Design review of the part built by this model. Coordinates are the model's own, in mm. Round coordinates to 2 decimals unless told otherwise and drop trailing zeros. Order: outer loops, then holes, each group sorted by start corner. A loop starts at its lowest first (then second) coordinate and runs counter-clockwise, first axis right, second up.
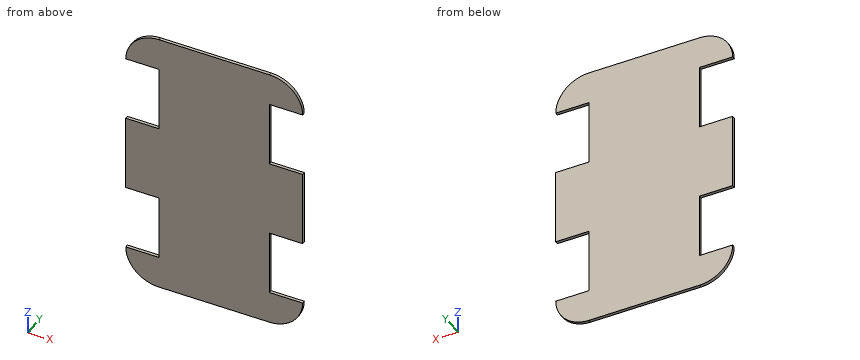
from build123d import *

# Parameters (mm, degrees)
BOSS_EXTRUDE1_DEPTH = 2.8


with BuildPart() as part:
    # Sketch1 → Boss-Extrude1 (new body)
    with BuildSketch(Plane(origin=(0, 0, 0), x_dir=(1, 0, 0), z_dir=(0, 1, 0))):
        with BuildLine():
            Line((0, 30), (30, 30))
            Line((30, 30), (30, 90))
            Line((30, 90), (0, 90))
            Line((0, 90), (0, 160))
            Line((0, 160), (30, 160))
            Line((30, 160), (30, 220))
            Line((30, 220), (0, 220))
            ThreePointArc((0, 220), (8.786796564, 241.213203436), (30, 250))
            Line((30, 250), (130, 250))
            ThreePointArc((130, 250), (151.213203436, 241.213203436), (160, 220))
            Line((160, 220), (130, 220))
            Line((130, 220), (130, 160))
            Line((130, 160), (160, 160))
            Line((160, 160), (160, 90))
            Line((160, 90), (130, 90))
            Line((130, 90), (130, 30))
            Line((130, 30), (160, 30))
            ThreePointArc((160, 30), (151.213203436, 8.786796564), (130, 0))
            Line((130, 0), (30, 0))
            ThreePointArc((30, 0), (8.786796564, 8.786796564), (0, 30))
        make_face()
    extrude(amount=BOSS_EXTRUDE1_DEPTH)


solid = part.part
1) Take a section at B-B on y = 2.2. Give the boundary of the cut face in (x, z).
Results:
outline: (0, -220) arc R30 ccw to (30, -250) - (130, -250) arc R30 ccw to (160, -220) - (130, -220) - (130, -160) - (160, -160) - (160, -90) - (130, -90) - (130, -30) - (160, -30) arc R30 ccw to (130, 0) - (30, 0) arc R30 ccw to (0, -30) - (30, -30) - (30, -90) - (0, -90) - (0, -160) - (30, -160) - (30, -220) - close
2) Take a section at A-A on x = 14. Give the boundary of the cut face in (y, z), plus the area to 3 significant figures.
Results:
outline: (0, -245.38) - (2.8, -245.38) - (2.8, -220) - (0, -220) - close; (0, -160) - (2.8, -160) - (2.8, -90) - (0, -90) - close; (0, -30) - (2.8, -30) - (2.8, -4.62) - (0, -4.62) - close
area: 338 mm2
3) To check wall thickness, follow line 1 along Z through (x, y) = (149, 1.4); line 2 along Z through (x, y) = (23, 0.6); line 3 along X through (y, z) = (2.35, -216.5). State the ranges of each line that lie inside material, in increasing order.
Results:
line 1: z = -243.22 to -220, -160 to -90, -30 to -6.78
line 2: z = -249.17 to -220, -160 to -90, -30 to -0.83
line 3: x = 30 to 130
4) Take a section at C-C on z = -211. Give the boundary of the cut face in (x, y), plus the area to 3 significant figures.
Results:
outline: (30, 0) - (130, 0) - (130, 2.8) - (30, 2.8) - close
area: 280 mm2
5) Take a section at D-D on z = -20.5. Give the boundary of the cut face in (x, y).
Results:
outline: (1.54, 0) - (158.46, 0) - (158.46, 2.8) - (1.54, 2.8) - close
6) Clearance check with flat-ended pins moving along their axes: P1, Ø0.8, axis at x = 15.5, y = 1.5, coming from the +Z side; P2, Ø1.4, axis at y = 2, z = -57.5, coming from the +X side; P3, Ø0.8, axis at x = 11, y = 1.5, coming from the +Z side. State where each tip first meets the part, or that it passes through.
Results:
P1: stops at z = -3.52
P2: stops at x = 130
P3: stops at z = -6.46
